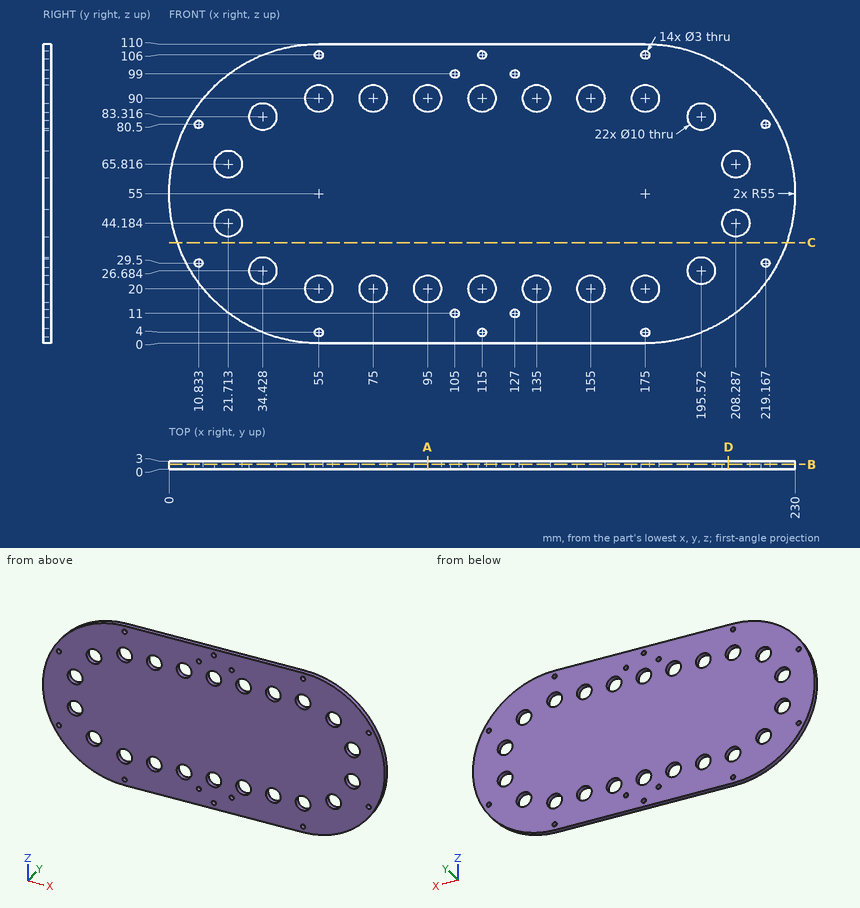
Could you check a few things on this drawing? It's one solid part, dimensions in mm from its lowest x, y, z. Give positions to 0.01 mm unless a question says otherwise; leave off trailing zeros. Loops run counter-clockwise (first coordinate to the right, second up) from the corner with the lowest first, then second, coordinate; pieces in that order, holes last. Notation, with made-up numbers: (65, 68.5) -> (81, 68.5) arc R15 ccw to (81, 77.5) -> close; hole circle Ø9 at (56, 18). An arc over 180 degrees is marked (long way). Answer as CSV lines item,"result". Start each with the question number.
(1) If we section it at C-C on z = 37: Write out the boundary of the cut face in (x, y).
(2) I need wall thicknesses on probe 1 along Z at (x, y) = (55, 0.95); probe 2 along Z at (x, y) = (105, 2.2); probe 3 along X at (y, z) = (0.1, 46.5) (1 decimal). Which ranges of each line are inside material? Lowest first, please.
(3) If we section it at A-A on x = 95: Write out the boundary of the cut face in (y, z).
(4) If we section it at B-B on y = 1.85: Count the separate pieces of the cut face and the enclosed holes in it, then the cut area to 3 significant figures.
(5) I'm going to push flat-ended pins straight in: pin 1 Ø13 at (x, z) = (21.71, 65.82) entering from +Y; pin 2 Ø2.5 at (x, z) = (127, 11) entering from -Y. Where does each tip first touch, or does it pass through?
(6) If we section it at D-D on x = 205.5: Write out the boundary of the cut face in (y, z) (1 decimal), then the cut area to 3 significant figures.
Computed:
1,outline,"(3.03, 0) -> (226.97, 0) -> (226.97, 3) -> (3.03, 3) -> close"
2,probe 1,"z = 0 to 2.5, 5.5 to 15, 25 to 85, 95 to 104.5, 107.5 to 110"
2,probe 2,"z = 0 to 9.5, 12.5 to 97.5, 100.5 to 110"
2,probe 3,"x = 0.7 to 17.3, 26.1 to 203.9, 212.7 to 229.3"
3,outline,"(0, 0) -> (3, 0) -> (3, 15) -> (0, 15) -> close; (0, 25) -> (3, 25) -> (3, 85) -> (0, 85) -> close; (0, 95) -> (3, 95) -> (3, 110) -> (0, 110) -> close"
4,separate pieces,"1"
4,enclosed holes,"36"
4,area,"20,900 mm2"
5,pin 1,"stops at y = 3"
5,pin 2,"passes through"
6,outline,"(0, 9.2) -> (3, 9.2) -> (3, 40) -> (0, 40) -> close; (0, 48.3) -> (3, 48.3) -> (3, 61.7) -> (0, 61.7) -> close; (0, 70) -> (3, 70) -> (3, 100.8) -> (0, 100.8) -> close"
6,area,"225 mm2"
